The model under review builds one solid part; all positions refer to its coordinate system, in mm. A direction names the side the tool comes from. Coordinates: 2 decimals unless noted, no trailing zeros. Order: outer loops, then holes, each group sorted by start corner. A loop starts at its lowest first (then second) coordinate and runs counter-clockwise, first axis right, second up. Notation, with made-up numbers: (-35.75, 84.5) - (-11.75, 84.5) arc R6 ccw to (-11.75, 90.5) - close; hole circle Ø11 at (-28, -12.5). An arc over 180 degrees is marked (long way). Answer in a Markdown table with one row per item.
```python
from build123d import *

# Parameters (mm, degrees)
ESQUISSE1_W      = 22
ESQUISSE1_H      = 22
EXTRUSION1_DEPTH = 374
ESQUISSE2_W      = 22
ESQUISSE2_H      = 22
EXTRUSION2_DEPTH = 60
ESQUISSE3_R      = 4.75
EXTRUSION3_DEPTH = 374


with BuildPart() as part:
    # Esquisse1 → Extrusion1 (new body)
    with BuildSketch(Plane.XY):
        with Locations((11, 11)):
            Rectangle(ESQUISSE1_W, ESQUISSE1_H)
    extrude(amount=EXTRUSION1_DEPTH)

    # Esquisse2 → Extrusion2 (add)
    with BuildSketch(Plane(origin=(22, 0, 0), x_dir=(0, 0, -1), z_dir=(1, 0, 0))):
        with Locations((-11, 11)):
            Rectangle(ESQUISSE2_W, ESQUISSE2_H)
        with Locations((-363, 11)):
            Rectangle(ESQUISSE2_W, ESQUISSE2_H)
        with Locations((-187, 11)):
            Rectangle(ESQUISSE2_W, ESQUISSE2_H)
    extrude(amount=EXTRUSION2_DEPTH)

    # Esquisse3 → Extrusion3 (cut)
    with BuildSketch(Plane.XY.offset(374)):
        with Locations((50, 11)):
            Circle(ESQUISSE3_R)
    extrude(amount=-EXTRUSION3_DEPTH, mode=Mode.SUBTRACT)


solid = part.part
```
Item 1: Clearance check with flat-ended pins moving along their axes: pin 1 Ø2 at (x, y) = (71, 8.5) entering from -Z; pin 2 Ø6 at (y, z) = (11.5, 240.5) entering from +X. State where each tip first meets the part, or that it passes through.
Check values:
| item | result |
|---|---|
| pin 1 | z = 0 |
| pin 2 | x = 22 |
Item 2: We need section A-A, the plane x = 50. Write out the cut boundary in (y, z).
Check values:
| item | result |
|---|---|
| outline | (0, 0) - (6.25, 0) - (6.25, 22) - (0, 22) - close; (0, 176) - (6.25, 176) - (6.25, 198) - (0, 198) - close; (0, 352) - (6.25, 352) - (6.25, 374) - (0, 374) - close; (15.75, 0) - (22, 0) - (22, 22) - (15.75, 22) - close; (15.75, 176) - (22, 176) - (22, 198) - (15.75, 198) - close; (15.75, 352) - (22, 352) - (22, 374) - (15.75, 374) - close |
Item 3: To check wall thickness, follow line 1 (Z direction, x = 40, y = 2.5); line 2 (Y direction, x = 50, z = 6); line 3 (X direction, y = 8.25, z = 136.5). State the ranges of each line that lie inside material, in increasing order. Write a range as from..to.
Check values:
| item | result |
|---|---|
| line 1 | 0..22, 176..198, 352..374 |
| line 2 | 0..6.25, 15.75..22 |
| line 3 | 0..22 |
Item 4: We need section D-D, the plane z = 265.5. Write out the cut boundary in (x, y).
Check values:
| item | result |
|---|---|
| outline | (0, 0) - (22, 0) - (22, 22) - (0, 22) - close |
Item 5: Tool access review of faces 1 (the face through (82, 11, 187)), 2 (the face through (52, 16, 22)): name each direction out of +Z, -Z, +X, -X, +Y, -Y from which nothing blocks a thin tool from reaching the whole face with its end or side.
Check values:
| item | result |
|---|---|
| face 1 | +Z, -Z, +X, +Y, -Y |
| face 2 | +X, +Y, -Y |
Item 6: We need section B-B, the plane y = 11. Write out the cut boundary in (x, z).
Check values:
| item | result |
|---|---|
| outline | (0, 0) - (45.25, 0) - (45.25, 22) - (22, 22) - (22, 176) - (45.25, 176) - (45.25, 198) - (22, 198) - (22, 352) - (45.25, 352) - (45.25, 374) - (0, 374) - close; (54.75, 0) - (82, 0) - (82, 22) - (54.75, 22) - close; (54.75, 176) - (82, 176) - (82, 198) - (54.75, 198) - close; (54.75, 352) - (82, 352) - (82, 374) - (54.75, 374) - close |
Item 7: Mouldability with a two-part tool opening along Y and no side actions: class faces 3 (the face through (52, 16, 352)), 4 (the face through (48.97, 6.363, 363.154)), 5 (the face through (13, 22, 231)) as +Y half, -Y half, draft (parallel to the pull), parting line (faces both ways), or undercut.
Check values:
| item | result |
|---|---|
| face 3 | draft |
| face 4 | undercut |
| face 5 | +Y half |
Item 8: We need section C-C, the plane x = 76. Write out the cut boundary in (y, z), then the cut area to 3 significant figures.
Check values:
| item | result |
|---|---|
| outline | (0, 0) - (22, 0) - (22, 22) - (0, 22) - close; (0, 176) - (22, 176) - (22, 198) - (0, 198) - close; (0, 352) - (22, 352) - (22, 374) - (0, 374) - close |
| area | 1,450 mm^2 |
